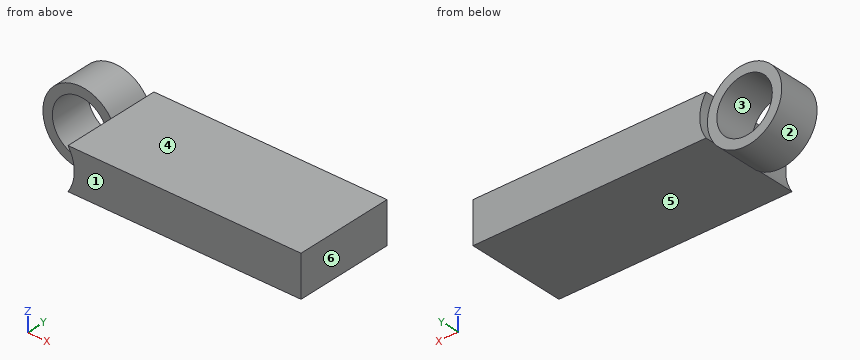
Autodesk Inventor part; units mm, degrees
ref_plane "YZ Plane" through (0, 0, 0) normal (1, 0, 0) x (0, 1, 0)
ref_plane "XZ Plane" through (0, 0, 0) normal (0, 1, 0) x (-1, 0, 0)
ref_plane "XY Plane" through (0, 0, 0) normal (0, 0, 1) x (1, 0, 0)
sketch "Sketch1" plane through (0, 0, 0) normal (0, 1, 0) x (-1, 0, 0)
  circle A0 centre (0, 0) radius 2.5
  circle A1 centre (0, 0) radius 3.35
  line L0 (-3.35, 0) -> (-15.85, 0) construction
  line L1 (-2.7822, 1.866) -> (-23.7822, 1.866)
  line L2 (-2.7822, -1.866) -> (-23.7822, -1.866)
  line L3 (-23.7822, -1.866) -> (-23.7822, 1.866)
  point P0 (0.2218, 3.3427)
  point P1 (0.2218, -3.3427)
  dimension "d0" = 5
  dimension "d1" = 6.7
  dimension "d2" = 12.5
  dimension "d12" = 21
extrude "Extrusion1" add sketch "Sketch1" along normal blind 3.7 contours A1
extrude "Extrusion3" add sketch "Sketch1" along normal mid plane 9 contours A1 L2 L3 L1
Input: part model. Units: mm. Frame: model coordinates. Face numbers are marked on the shaded views. A direction names the side the tool comes from. Coordinates: 2 decimals unless noted, no trailing zeros. Write each loop counter-clockwise with the first axis right and the second up, starting at its lowest first coordinate (ties: lowest second). Pieces come first, ordered by that corner, then holes. Notation, with made-up numbers: (28.5, 13) - (73.5, 13) arc R16 ccw to (73.5, 22) - close; hole circle Ø3 at (-14.75, 70). An arc over 180 degrees is marked (long way). Put each result on its own line as item: value. Start each with the question number.
1) Contact query for flat-ended pins moving along their axis: pin 1 (2.5 mm diameter, centred on x = 18.5, y = -0.5, fed in from +Z); pin 2 (3.5 mm diameter, centred on x = 1, z = -1, fed in from +Y); pin 3 (1.5 mm diameter, centred on x = 1, y = -0.5, fed in from -Z). Output: stop coordinate, or through.
2) Cut plane A-A (x = 0). Return the cut outline in (y, z).
3) Cut plane D-D (y = -3.25). Return the cut outline in (x, z), plus the area to 3 significant figures.
4) Cut plane C-C (y = 0.5). Return the cut outline in (x, z).
5) Cut plane B-B (z = 0). Return the cut outline in (x, y).
6) Mould query, pull axis X, two halves, no side actions, for the marked faces 1, 2 and 3. Classes: pulls with the +X half, pulls with the -X half, needs draft (parallel to the pull), parting line crosses it, or undercut.
7) Ray query, L1, parallel to Z at x = 0, y = 1.9; L2, parallel to Z at x = 17.75, y = -0.5; L3, parallel to X at y = 3, z = 1. Return the intervals inside material, ascending.
8) Reachability of the marked faces 4, 5 and 6 from +Z, -Z, +X, -X, +Y, -Y: full face, straight path, thin tool, end or side. Return the list, or none.
Resolved:
1. pin 1: stops at z = 1.87
1. pin 2: stops at y = 3.7
1. pin 3: stops at z = -3.32
2. outline: (0, -3.35) - (3.7, -3.35) - (3.7, -2.5) - (0, -2.5) - close; (0, 2.5) - (3.7, 2.5) - (3.7, 3.35) - (0, 3.35) - close
3. outline: (2.78, -1.87) - (23.78, -1.87) - (23.78, 1.87) - (2.78, 1.87) arc R3.35 cw to start
3. area: 76.9 mm2
4. outline: (2.78, -1.87) - (23.78, -1.87) - (23.78, 1.87) - (2.78, 1.87) arc R3.35 ccw (long way) to start; hole circle Ø5 at (0, 0)
5. outline: (-3.35, 0) - (-2.5, 0) - (-2.5, 3.7) - (-3.35, 3.7) - close; (2.5, 0) - (3.35, 0) - (3.35, -4.5) - (23.78, -4.5) - (23.78, 4.5) - (3.35, 4.5) - (3.35, 3.7) - (2.5, 3.7) - close
6. face 1: needs draft
6. face 2: parting line crosses it
6. face 3: undercut
7. L1: z = -3.35 to -2.5, 2.5 to 3.35
7. L2: z = -1.87 to 1.87
7. L3: x = -3.2 to -2.29, 2.29 to 23.78
8. face 4: +Z, +X, +Y, -Y
8. face 5: -Z, +X, +Y, -Y
8. face 6: +Z, -Z, +X, +Y, -Y
